```python
from build123d import *

# Parameters (mm, degrees)
SKETCH2_R           = 5
SKETCH2_R_2         = 1.5
BOSS_EXTRUDE1_DEPTH = 3
SKETCH3_W           = 46
SKETCH3_H           = 3
BOSS_EXTRUDE2_DEPTH = 27
CUT_EXTRUDE1_DEPTH  = 52.51698749
FILLET1_R           = 1
FILLET2_R           = 1


with BuildPart() as part:
    # Sketch2 → Boss-Extrude1 (new body)
    with BuildSketch(Plane(origin=(0, 0, 0), x_dir=(1, 0, 0), z_dir=(0, 1, 0))):
        with BuildLine():
            Line((-22, 19), (22, 19))
            ThreePointArc((22, 19), (22.707106781, 18.707106781), (23, 18))
            Line((23, 18), (23, -19))
            Line((23, -19), (-23, -19))
            Line((-23, -19), (-23, 18))
            ThreePointArc((-23, 18), (-22.707106781, 18.707106781), (-22, 19))
        make_face()
        with Locations(Location((8, 3, 0), (0, 0, 270))):
            Circle(SKETCH2_R, mode=Mode.SUBTRACT)
        with Locations(Location((-8, 3, 0), (0, 0, 90))):
            Circle(SKETCH2_R, mode=Mode.SUBTRACT)
        with Locations(Location((-16.5, 12, 0), (0, 0, 270))):
            Circle(SKETCH2_R_2, mode=Mode.SUBTRACT)
        with Locations(Location((-16.5, -6, 0), (0, 0, 90))):
            Circle(SKETCH2_R_2, mode=Mode.SUBTRACT)
        with Locations(Location((16.5, -6, 0), (0, 0, 270))):
            Circle(SKETCH2_R_2, mode=Mode.SUBTRACT)
        with Locations(Location((16.5, 12, 0), (0, 0, 90))):
            Circle(SKETCH2_R_2, mode=Mode.SUBTRACT)
    extrude(amount=BOSS_EXTRUDE1_DEPTH)

    # Sketch3 → Boss-Extrude2 (add)
    with BuildSketch(Plane(origin=(0, 3, 0), x_dir=(1, 0, 0), z_dir=(0, 1, 0))):
        with Locations((0, -17.5)):
            Rectangle(SKETCH3_W, SKETCH3_H)
    extrude(amount=BOSS_EXTRUDE2_DEPTH)

    # Sketch4 → Cut-Extrude1 (cut, through all)
    with BuildSketch(Plane(origin=(0, 0, 16), x_dir=(-1, 0, 0), z_dir=(0, 0, -1))):
        with BuildLine():
            Line((-17, 23.5), (-17, 9.5))
            ThreePointArc((-17, 9.5), (-15, 7.5), (-13, 9.5))
            Line((-13, 9.5), (-13, 23.5))
            ThreePointArc((-13, 23.5), (-15, 25.5), (-17, 23.5))
        make_face()
        with BuildLine():
            Line((13, 23.5), (13, 9.5))
            ThreePointArc((13, 9.5), (15, 7.5), (17, 9.5))
            Line((17, 9.5), (17, 23.5))
            ThreePointArc((17, 23.5), (15, 25.5), (13, 23.5))
        make_face()
    extrude(amount=-CUT_EXTRUDE1_DEPTH, mode=Mode.SUBTRACT)

    # Fillet1
    fillet1_edges = [part.edges().sort_by_distance(p)[0] for p in [
        (-23, 30, 17.5),
        (23, 30, 17.5),
    ]]
    fillet(fillet1_edges, radius=FILLET1_R)

    # Fillet2
    fillet2_edges = [part.edges().sort_by_distance(p)[0] for p in [
        (0, 0, 19),
    ]]
    fillet(fillet2_edges, radius=FILLET2_R)


solid = part.part
```
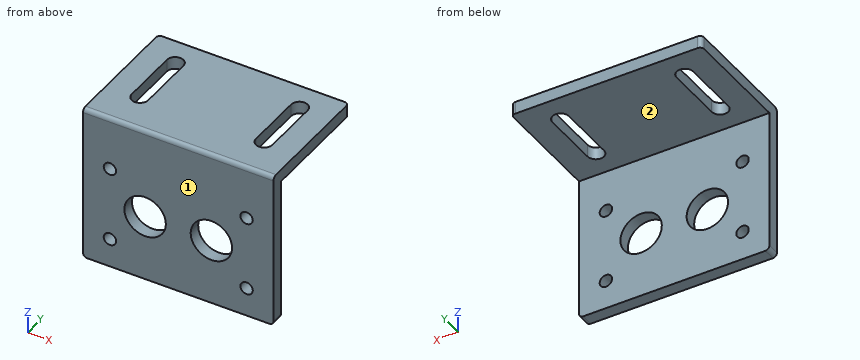
The listing builds one solid part. Answer for the finished solid, in the listing's coordinates (mm). Face numbers are marked on the shaded views. A direction names the side the tool comes from. Round coordinates to 2 decimals unless told otherwise and drop trailing zeros. Order: outer loops, then holes, each group sorted by start corner. A loop starts at its lowest first (then second) coordinate and runs counter-clockwise, first axis right, second up. Notation, with made-up numbers: (-13.75, -32) -> (-2.75, -32) arc R20 ccw to (-2.75, -7) -> close; hole circle Ø4 at (36, -7). An arc over 180 degrees is marked (long way). Answer as CSV lines item,"result".
Q1. A cutting plane is placed at C-C on x = 1. Determine the outline of the cut face in (y, z).
Computed values:
outline,"(0, -19) -> (3, -19) -> (3, 16) -> (30, 16) -> (30, 19) -> (1, 19) arc R1 ccw to (0, 18) -> close"
Q2. Given pin 1 (8 mm diameter, centred on x = 12.5, z = -6, fed in from +Y); pin 2 (1 mm diameter, centred on x = -4, y = 11.5, fed in from -Z); pin 3 (2.5 mm diameter, centred on x = 16.5, z = 6, fed in from +Y), each flat-ended and moving along its own axis, determine where each tip first touches the part or whether it passes through.
Computed values:
pin 1,"stops at y = 3"
pin 2,"stops at z = 16"
pin 3,"passes through"
Q3. A cutting plane is placed at D-D on z = -12. Determine the outline of the cut face in (x, y).
Computed values:
outline,"(-23, 0) -> (-18, 0) -> (-18, 3) -> (-23, 3) -> close; (-15, 0) -> (15, 0) -> (15, 3) -> (-15, 3) -> close; (18, 0) -> (23, 0) -> (23, 3) -> (18, 3) -> close"
Q4. Consider line 1 (X direction, y = 1, z = -3); line 2 (X direction, y = 1.15, z = -12); line 3 (Z direction, x = 8, y = 13). Determine where each line is inside the solid, lowest interval first. Write a range as from..to.
Computed values:
line 1,"x = -23..-13, -3..3, 13..23"
line 2,"x = -23..-18, -15..15, 18..23"
line 3,"z = 16..19"
Q5. Which of the six approach directions +Z, -Z, +X, -X, +Y, -Y give full straight-line access (tool end or side, diameter ignored) to the marked faces 1 and 2?
Computed values:
face 1,"+Z, -Z, +X, -X, -Y"
face 2,"-Z, +X, -X, +Y"
Q6. A cutting plane is placed at A-A on z = -3. Determine the outline of the cut face in (x, y).
Computed values:
outline,"(-23, 0) -> (-13, 0) -> (-13, 3) -> (-23, 3) -> close; (-3, 0) -> (3, 0) -> (3, 3) -> (-3, 3) -> close; (13, 0) -> (23, 0) -> (23, 3) -> (13, 3) -> close"
Q7. A cutting plane is placed at B-B on x = -8. Determine the outline of the cut face in (y, z).
Computed values:
outline,"(0, -19) -> (3, -19) -> (3, -8) -> (0, -8) -> close; (0, 2) -> (3, 2) -> (3, 16) -> (30, 16) -> (30, 19) -> (1, 19) arc R1 ccw to (0, 18) -> close"
